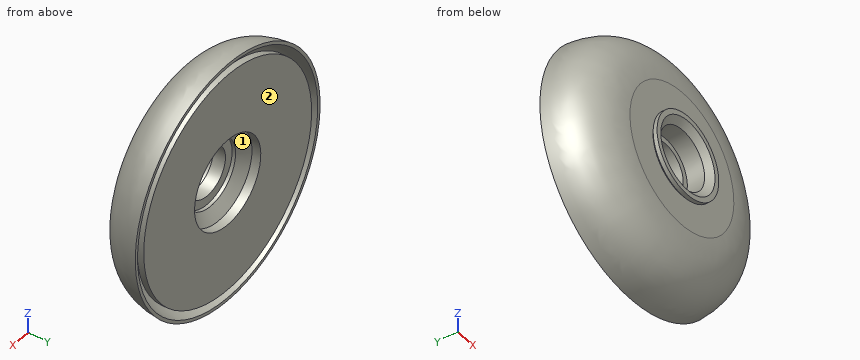
from build123d import *


with BuildPart() as part:
    # Sketch1 → Revolve1 (revolve)
    with BuildSketch(Plane.XY, mode=Mode.PRIVATE) as revolve1_sk:
        with BuildLine():
            Line((-21.8, 5.207082814), (-8.6, 5.207082814))
            Line((-8.6, 5.207082814), (-8.6, 3.487716788))
            Line((-8.6, 3.487716788), (-6.45, 1.893195372))
            Line((-6.45, 1.893195372), (-6.45, 1.207082814))
            Line((-6.45, 1.207082814), (-4.725, 1.207082814))
            Line((-4.725, 1.207082814), (-4.725, -1.207082814))
            Line((-4.725, -1.207082814), (-5.792193517, -1.207082814))
            Line((-5.792193517, -1.207082814), (-5.792193517, -4.58565461))
            Line((-5.792193517, -4.58565461), (-7.039346549, -5.692917186))
            Line((-7.039346549, -5.692917186), (-8.009354463, -5.692917186))
            Line((-8.009354463, -5.692917186), (-8.009354463, -4.922332057))
            Line((-8.009354463, -4.922332057), (-7.484167863, -4.512624738))
            Line((-7.484167863, -4.512624738), (-13.491490452, -4.512624738))
            add(Edge.make_bspline(
                [(-24, 5.207082814), (-23.362064214, -4.252005312), (-13.491490452, -4.512624738)],
                knots=[0, 0, 0, 1, 1, 1], degree=2))
            Line((-24, 5.207082814), (-23.4, 5.207082814))
            add(Edge.make_bspline(
                [(-12.616940425, -3.912624738), (-22.084892945, -3.918102421), (-23.4, 5.207082814)],
                knots=[0, 0, 0, 1, 1, 1], degree=2))
            Line((-12.616940425, -3.912624738), (-11, -3.912624738))
            Line((-11, -3.912624738), (-11, 3.907082814))
            Line((-11, 3.907082814), (-21.8, 3.907082814))
            Line((-21.8, 3.907082814), (-21.8, 5.207082814))
        make_face()
    revolve(revolve1_sk.sketch.rotate(Axis((0, 24.52235385, 0), (0, -1, 0)), 270), axis=Axis((0, 24.52235385, 0), (0, -1, 0)))


solid = part.part
Could you check a few things on this model? Use its own coordinates, in mm. Face numbers are marked on the shaded views. Give positions to 0.01 mm unless a question says otherwise; leave off trailing zeros. Answer in a Markdown table with one row per item. Add a question column.
Item 1: We'd pull the mould along X, two halves only. Please class the marked faces 1 and 2: pulls with the +X half, pulls with the -X half, needs draft (parallel to the pull), parting line crosses it, or undercut.
Item 2: Please list where these lines run through material, in increasing order: probe 1 along Z at (x, y) = (8, -1.25); probe 2 along X at (y, z) = (2, -0.5); probe 3 along X at (y, z) = (2, -10).
Item 3: I'm going to push flat-ended pins straight in: P1, Ø3, axis at x = -7, y = -3, coming from the -Z side; P2, Ø4, axis at x = 0.5, z = 3, coming from the +Y side; P3, Ø6, axis at y = -1, z = -2.5, coming from the -X side; P4, Ø3, axis at x = -13, z = 18.5, coming from the +Y side. Where does each tip first touch, or does it pass through?
Item 4: Imagine slicing it at A-A (y = -2.25). Count the separate pieces of the cut face and the enclosed holes in it, and give its area (3 significant figures).
Result:
| question | item | result |
|---|---|---|
| 1 | face 1 | undercut |
| 1 | face 2 | needs draft |
| 2 | probe 1 | -20.2 to -18.84, -7.55 to 7.55, 18.84 to 20.2 |
| 2 | probe 2 | -23.44 to -22.57, -10.99 to -6.58, 6.58 to 10.99, 22.57 to 23.44 |
| 2 | probe 3 | -21.2 to -20.24, -4.58 to 4.58, 20.24 to 21.2 |
| 3 | P1 | z = -20.42 |
| 3 | P2 | y = 1.21 |
| 3 | P3 | x = -23.35 |
| 3 | P4 | y = 5.21 |
| 4 | separate pieces | 2 |
| 4 | enclosed holes | 2 |
| 4 | area | 462 mm2 |
